```python
from build123d import *

# Parameters (mm, degrees)
SKETCH_1_R                       = 2.75
SKETCH_1_R_2                     = 0.85
EXTRUDE_1_DEPTH                  = 3.4
SKETCH_2_R                       = 0.45
EXTRUDE_2_DEPTH                  = 1
SKETCH_3_R                       = 0.45
CUT_EXTRUDE_1_DEPTH              = 4.4
HOLE_WIZARD_1_3_1_3_1_AT_2_COUNT = 2
HOLE_WIZARD_1_3_1_3_1_AT_2_PITCH = 5.656854249
HOLE_WIZARD_1_3_1_3_1_AT_3_COUNT = 2
HOLE_WIZARD_1_3_1_3_1_AT_3_PITCH = 8


with BuildPart() as part:
    # Эскиз1 → Бобышка-Вытянуть1 (new body)
    with BuildSketch(Plane(origin=(0, 0, 0), x_dir=(1, 0, 0), z_dir=(0, 1, 0))):
        Circle(SKETCH_1_R)
        Circle(SKETCH_1_R_2, mode=Mode.SUBTRACT)
    extrude(amount=EXTRUDE_1_DEPTH)

    # Эскиз2 → Бобышка-Вытянуть2 (add)
    with BuildSketch(Plane(origin=(0, 3.4, 0), x_dir=(1, 0, 0), z_dir=(0, 1, 0))):
        with BuildLine():
            Line((6.9, 1.8), (2.079062289, 1.8))
            ThreePointArc((2.079062289, 1.8), (2.75, 0), (2.079062289, -1.8))
            Line((2.079062289, -1.8), (6.9, -1.8))
            ThreePointArc((6.9, -1.8), (8.7, 0), (6.9, 1.8))
        make_face()
        with Locations((6.9, 0)):
            Circle(SKETCH_2_R, mode=Mode.SUBTRACT)
        with BuildLine():
            ThreePointArc((-1.8, 2.079062289), (0, 2.75), (1.8, 2.079062289))
            Line((1.8, 2.079062289), (1.8, 6.9))
            ThreePointArc((1.8, 6.9), (0, 8.7), (-1.8, 6.9))
            Line((-1.8, 6.9), (-1.8, 2.079062289))
        make_face()
        with Locations((0, 6.9)):
            Circle(SKETCH_2_R, mode=Mode.SUBTRACT)
        with BuildLine():
            Line((1.8, -6.9), (1.8, -2.079062289))
            ThreePointArc((1.8, -2.079062289), (0, -2.75), (-1.8, -2.079062289))
            Line((-1.8, -2.079062289), (-1.8, -6.9))
            ThreePointArc((-1.8, -6.9), (0, -8.7), (1.8, -6.9))
        make_face()
        with Locations((0, -6.9)):
            Circle(SKETCH_2_R, mode=Mode.SUBTRACT)
        with BuildLine():
            ThreePointArc((-2.079062289, -1.8), (-2.75, 0), (-2.079062289, 1.8))
            Line((-2.079062289, 1.8), (-6.9, 1.8))
            ThreePointArc((-6.9, 1.8), (-8.7, 0), (-6.9, -1.8))
            Line((-6.9, -1.8), (-2.079062289, -1.8))
        make_face()
        with Locations((-6.9, 0)):
            Circle(SKETCH_2_R, mode=Mode.SUBTRACT)
    extrude(amount=-EXTRUDE_2_DEPTH)

    # Эскиз3 → Вырез-Вытянуть1 (cut, through all)
    with BuildSketch(Plane(origin=(0, 3.4, 0), x_dir=(1, 0, 0), z_dir=(0, 1, 0))):
        with BuildLine():
            Line((6.9, 1.8), (5, 1.8))
            Line((5, 1.8), (5, -1.8))
            Line((5, -1.8), (6.9, -1.8))
            ThreePointArc((6.9, -1.8), (8.7, 0), (6.9, 1.8))
        make_face()
        with Locations((6.9, 0)):
            Circle(SKETCH_3_R, mode=Mode.SUBTRACT)
        with BuildLine():
            Line((1.8, -5), (-1.8, -5))
            Line((-1.8, -5), (-1.8, -6.9))
            ThreePointArc((-1.8, -6.9), (0, -8.7), (1.8, -6.9))
            Line((1.8, -6.9), (1.8, -5))
        make_face()
        with Locations((0, -6.9)):
            Circle(SKETCH_3_R, mode=Mode.SUBTRACT)
        with BuildLine():
            Line((-1.8, 6.9), (-1.8, 5))
            Line((-1.8, 5), (1.8, 5))
            Line((1.8, 5), (1.8, 6.9))
            ThreePointArc((1.8, 6.9), (0, 8.7), (-1.8, 6.9))
        make_face()
        with Locations((0, 6.9)):
            Circle(SKETCH_3_R, mode=Mode.SUBTRACT)
    extrude(amount=-CUT_EXTRUDE_1_DEPTH, mode=Mode.SUBTRACT)

    # Эскиз4 → Диаметр отверстия Ø1.3 (1.3)1 (revolve, cut)
    with BuildSketch(Plane(origin=(0, 2.4, -4), x_dir=(0, 0, -1), z_dir=(1, 0, 0))):
        Polygon((0, 0), (0, 1), (0.675, 1), (0.65, 0.975), (0.65, 0.025), (0.675, 0), align=None)
    hole_wizard_1_3_1_3_1 = revolve(axis=Axis((0, -3.95, -4), (0, 1, 0)), mode=Mode.SUBTRACT)

    # Диаметр отверстия Ø1.3 (1.3)1 at 2: Диаметр отверстия Ø1.3 (1.3)1 ×2
    with Locations(*[Vector(0.707106781, 0, 0.707106781) * (i * HOLE_WIZARD_1_3_1_3_1_AT_2_PITCH) for i in range(1, HOLE_WIZARD_1_3_1_3_1_AT_2_COUNT)]):
        add(hole_wizard_1_3_1_3_1, mode=Mode.SUBTRACT)

    # Диаметр отверстия Ø1.3 (1.3)1 at 3: Диаметр отверстия Ø1.3 (1.3)1 ×2
    with Locations(*[(0, 0, i * HOLE_WIZARD_1_3_1_3_1_AT_3_PITCH) for i in range(1, HOLE_WIZARD_1_3_1_3_1_AT_3_COUNT)]):
        add(hole_wizard_1_3_1_3_1, mode=Mode.SUBTRACT)


solid = part.part
```
Build history of the part. All positions in model axes, mm. A direction names the side the tool comes from. Round coordinates to 2 decimals unless told otherwise and drop trailing zeros. Write each loop counter-clockwise with the first axis right and the second up, starting at its lowest first coordinate (ties: lowest second). Pieces come first, ordered by that corner, then holes. Notation, with made-up numbers: (-22, 65) - (-8, 65) arc R27 ccw to (-8, 83) - close; hole circle Ø4 at (-34.75, 67). An arc over 180 degrees is marked (long way). Write each question's results on one line, items separated by ' | '. Start each with the question number.
Item 1: Mould opens along X. For faces 1 (the face through (-0.2, 2.89, -4.62)), 2 (the face through (-2.027, 1.298, -1.859)), 3 (the face through (0, 3, -5)) say: pulls with the +X half, pulls with the -X half, needs draft (parallel to the pull), parting line crosses it, or undercut.
Item 2: Saw through at B-B (y = 2.85). Write the cut outline in (x, z), and give its area (3 significant figures).
Item 3: Saw through at C-C (x = 0). Write the cut outline in (y, z) (3 decimals), and give its area (3 significant figures).
Item 4: Drop flat-ended pins along their axis: P1, Ø0.5, axis at y = 2.5, z = 3.5, coming from the -X side; P2, Ø1.2, axis at x = 0, z = 4, coming from the -Y side; P3, Ø1.1, axis at x = -6, z = 0, coming from the -Y side; P4, Ø0.5, axis at x = 4, y = 3, coming from the +Z side. Give the stop position or say it passes through.
Item 5: Wall check: L1, parallel to X at y = 3.05, z = 0; L2, parallel to X at y = 2.5, z = -0.5; L3, parallel to Z at x = 0, y = 0.8. Give the ranges that are in metal, low to high. Write a range as [from, to].
Item 6: Saw through at D-D (x = 4). Write the cut outline in (y, z) (3 decimals).
Item 7: Which spindle directions (+Z, -Z, +X, -X, +Y, -Y) get a long thin tool onto all of the face, cutting with end or side? Do faces 4 (the face through (4, 3, -1.8)), 5 (the face through (-5, 3, 1.8)), 6 (the face through (-4, 3, -1.8)), 7 (the face through (4, 3, 1.8)). Say none if no direction does.
Item 8: Saw through at A-A (z = 0). Write the cut outline in (x, y) (3 decimals), and give its area (3 significant figures).
Results are:
1) face 1: undercut | face 2: parting line crosses it | face 3: needs draft
2) outline: (-6.9, -1.8) - (-2.08, -1.8) arc R2.75 ccw to (-1.8, -2.08) - (-1.8, -5) - (1.8, -5) - (1.8, -2.08) arc R2.75 ccw to (2.08, -1.8) - (5, -1.8) - (5, 1.8) - (2.08, 1.8) arc R2.75 ccw to (1.8, 2.08) - (1.8, 5) - (-1.8, 5) - (-1.8, 2.08) arc R2.75 ccw to (-2.08, 1.8) - (-6.9, 1.8) arc R1.8 ccw to start; hole circle Ø0.9 at (-6.9, 0); hole circle Ø1.7 at (0, 0); hole circle Ø1.3 at (0, -4); hole circle Ø1.3 at (0, 4); hole circle Ø1.3 at (4, 0) | area: 64.2 mm²
3) outline: (0, -2.75) - (2.4, -2.75) - (2.4, -3.325) - (2.425, -3.35) - (3.375, -3.35) - (3.4, -3.325) - (3.4, -0.85) - (0, -0.85) - close; (0, 0.85) - (3.4, 0.85) - (3.4, 3.325) - (3.375, 3.35) - (2.425, 3.35) - (2.4, 3.325) - (2.4, 2.75) - (0, 2.75) - close; (2.4, -5) - (3.4, -5) - (3.4, -4.675) - (3.375, -4.65) - (2.425, -4.65) - (2.4, -4.675) - close; (2.4, 4.675) - (2.425, 4.65) - (3.375, 4.65) - (3.4, 4.675) - (3.4, 5) - (2.4, 5) - close | area: 14.8 mm²
4) P1: stops at x = -1.8 | P2: passes through | P3: stops at y = 2.4 | P4: stops at z = 1.8
5) L1: x = [-8.7, -7.35], [-6.45, -0.85], [0.85, 3.35], [4.65, 5] | L2: x = [-8.63, -0.69], [0.69, 3.58], [4.42, 5] | L3: z = [-2.75, -0.85], [0.85, 2.75]
6) outline: (2.4, -1.8) - (3.4, -1.8) - (3.4, -0.675) - (3.375, -0.65) - (2.425, -0.65) - (2.4, -0.675) - close; (2.4, 0.675) - (2.425, 0.65) - (3.375, 0.65) - (3.4, 0.675) - (3.4, 1.8) - (2.4, 1.8) - close
7) face 4: -Z, +X, +Y, -Y | face 5: +Z, -X, +Y, -Y | face 6: -Z, -X, +Y, -Y | face 7: +Z, +X, +Y, -Y
8) outline: (-8.7, 2.4) - (-7.35, 2.4) - (-7.35, 3.4) - (-8.7, 3.4) - close; (-6.45, 2.4) - (-2.75, 2.4) - (-2.75, 0) - (-0.85, 0) - (-0.85, 3.4) - (-6.45, 3.4) - close; (0.85, 0) - (2.75, 0) - (2.75, 2.4) - (3.325, 2.4) - (3.35, 2.425) - (3.35, 3.375) - (3.325, 3.4) - (0.85, 3.4) - close; (4.65, 2.425) - (4.675, 2.4) - (5, 2.4) - (5, 3.4) - (4.675, 3.4) - (4.65, 3.375) - close | area: 18.9 mm²
